Autodesk Inventor part; units mm, degrees
ref_plane "YZ Plane" through (0, 0, 0) normal (1, 0, 0) x (0, 1, 0)
ref_plane "XZ Plane" through (0, 0, 0) normal (0, 1, 0) x (-1, 0, 0)
ref_plane "XY Plane" through (0, 0, 0) normal (0, 0, 1) x (1, 0, 0)
sketch "Sketch1" plane through (0, 0, 0) normal (0, 0, 1) x (1, 0, 0)
  line L0 (-96.7048, 41.9035) -> (-96.7048, -42.0965)
  line L1 (-96.7048, -42.0965) -> (-72.3448, -42.0965)
  line L2 (-72.3448, -42.0965) -> (-72.3448, -36.0115)
  line L3 (-72.3448, -36.0115) -> (-48.7048, -36.0115)
  line L4 (-48.7048, -36.0115) -> (-48.7048, -42.0965)
  line L5 (-48.7048, -42.0965) -> (-24.3448, -42.0965)
  line L6 (-0.7048, -42.0965) -> (23.6552, -42.0965)
  line L7 (47.2952, -42.0965) -> (71.6552, -42.0965)
  line L8 (71.6552, -42.0965) -> (71.6552, -36.0115)
  line L9 (71.6552, -36.0115) -> (95.2952, -36.0115)
  line L10 (95.2952, -36.0115) -> (95.2952, 35.8185)
  line L11 (95.2952, 35.8185) -> (71.6552, 35.8185)
  line L12 (71.6552, 35.8185) -> (71.6552, 41.9035)
  line L13 (71.6552, 41.9035) -> (47.2952, 41.9035)
  line L14 (47.2952, 41.9035) -> (47.2952, 35.8185)
  line L15 (47.2952, 35.8185) -> (23.6552, 35.8185)
  line L16 (23.6552, 35.8185) -> (23.6552, 41.9035)
  line L17 (23.6552, 41.9035) -> (-0.7048, 41.9035)
  line L18 (-0.7048, 41.9035) -> (-0.7048, 35.8185)
  line L19 (-0.7048, 35.8185) -> (-24.3448, 35.8185)
  line L20 (-24.3448, 35.8185) -> (-24.3448, 41.9035)
  line L21 (-24.3448, 41.9035) -> (-48.7048, 41.9035)
  line L22 (-48.7048, 41.9035) -> (-48.7048, 35.8185)
  line L23 (-48.7048, 35.8185) -> (-72.3448, 35.8185)
  line L24 (-72.3448, 35.8185) -> (-72.3448, 41.9035)
  line L25 (-72.3448, 41.9035) -> (-96.7048, 41.9035)
  line L26 (-24.3448, -42.0965) -> (-24.3448, -36.0115)
  line L27 (-24.3448, -36.0115) -> (-0.7048, -36.0115)
  line L28 (-0.7048, -36.0115) -> (-0.7048, -42.0965)
  line L29 (23.6552, -42.0965) -> (23.6552, -36.0115)
  line L30 (23.6552, -36.0115) -> (47.2952, -36.0115)
  line L31 (47.2952, -36.0115) -> (47.2952, -42.0965)
  point P0 (0, 0)
  dimension "d0" = 84
  dimension "d1" = 24.36
  dimension "d2" = 23.64
  dimension "d3" = 24.36
  dimension "d5" = 24.36
  dimension "d8" = 23.64
  dimension "d9" = 71.83
  dimension "d10" = 23.64
  dimension "d11" = 6.085
  dimension "d12" = 6.085
  dimension "d13" = 6.085
  dimension "d14" = 24.36
  dimension "d15" = 23.64
  dimension "d16" = 24.36
  dimension "d17" = 23.64
  dimension "d18" = 24.36
  dimension "d19" = 23.64
  dimension "d20" = 24.36
  dimension "d21" = 23.64
  dimension "d22" = 23.64
extrude "Extrusion1" add sketch "Sketch1" against normal blind 3.25
sketch "Sketch2" plane through (0, 0, 0) normal (0, 0, 1) x (1, 0, 0)
  line L0 (-92.5348, 22.4285) -> (-92.5348, -22.6215)
  line L1 (-92.5348, -22.6215) -> (-88.4348, -22.6215)
  line L2 (-88.4348, -22.6215) -> (-88.4348, 22.4285)
  line L3 (-88.4348, 22.4285) -> (-92.5348, 22.4285)
  line L4 (-96.7048, 41.9035) -> (-96.7048, -42.0965)
  line L5 (-72.3448, 41.9035) -> (-96.7048, 41.9035)
  line L6 (-85.7648, 13.0835) -> (-85.7648, -13.2765)
  line L7 (-85.7648, -13.2765) -> (-58.5248, -13.2765)
  line L8 (-58.5248, -13.2765) -> (-58.5248, 13.0835)
  line L9 (-58.5248, 13.0835) -> (-85.7648, 13.0835)
  line L10 (-54.5548, 31.9735) -> (-54.5548, -32.1665)
  line L11 (-54.5548, -32.1665) -> (-41.9148, -32.1665)
  line L12 (-41.9148, -32.1665) -> (-41.9148, 31.9735)
  line L13 (-41.9148, 31.9735) -> (-54.5548, 31.9735)
  line L14 (-24.3448, 41.9035) -> (-48.7048, 41.9035)
  line L15 (-29.3448, 21.4335) -> (-29.3448, -21.6265)
  line L16 (-29.3448, -21.6265) -> (65.1152, -21.6265)
  line L17 (65.1152, -21.6265) -> (65.1152, 21.4335)
  line L18 (65.1152, 21.4335) -> (-29.3448, 21.4335)
  line L19 (73.8852, 31.9735) -> (73.8852, -32.1665)
  line L20 (73.8852, -32.1665) -> (86.5252, -32.1665)
  line L21 (86.5252, -32.1665) -> (86.5252, 31.9735)
  line L22 (71.6552, 35.8185) -> (95.2952, 35.8185)
  line L23 (86.5252, 31.9735) -> (73.8852, 31.9735)
  line L24 (95.2952, -36.0115) -> (95.2952, 35.8185)
  point P0 (0, 0)
  dimension "d25" = 4.17
  dimension "d26" = 4.1
  dimension "d27" = 45.05
  dimension "d28" = 19.475
  dimension "d29" = 10.94
  dimension "d30" = 26.36
  dimension "d31" = 27.24
  dimension "d32" = 42.15
  dimension "d33" = 28.82
  dimension "d34" = 64.14
  dimension "d35" = 12.64
  dimension "d36" = 9.93
  dimension "d37" = 67.36
  dimension "d38" = 43.06
  dimension "d39" = 94.46
  dimension "d40" = 20.47
  dimension "d41" = 64.14
  dimension "d42" = 12.64
  dimension "d43" = 3.845
  dimension "d44" = 8.77
extrude "Extrusion2" cut sketch "Sketch2" against normal blind 4
sketch "Sketch3" plane through (0, 0, 0) normal (0, 0, 1) x (1, 0, 0)
  line L0 (-121.7905, 18.4035) -> (-90.4348, 18.4035)
  line L1 (-90.4348, 18.4035) -> (-90.4348, -18.5965)
  line L2 (-88.4348, 22.4285) -> (-88.4348, -22.6215)
  line L3 (-90.4348, -18.5965) -> (-121.7905, -18.5965)
  line L4 (-121.7905, -18.5965) -> (-121.7905, 18.4035)
  line L5 (-72.3448, 41.9035) -> (-96.7048, 41.9035)
  point P0 (0, 0)
  dimension "d47" = 37
  dimension "d48" = 23.5
  dimension "d49" = 2
extrude "Extrusion3" cut sketch "Sketch3" against normal blind 4
sketch "Sketch9" plane through (0, 0, 0) normal (0, 0, 1) x (1, 0, 0)
  line L0 (-92.5348, 28.4035) -> (-92.5348, -28.5965)
  line L1 (-92.5348, -28.5965) -> (-159.1348, -28.5965)
  line L2 (-159.1348, -28.5965) -> (-159.1348, 28.4035)
  line L3 (-159.1348, 28.4035) -> (-92.5348, 28.4035)
  line L4 (-92.5348, 18.4035) -> (-92.5348, 22.4285)
  line L5 (-72.3448, 41.9035) -> (-96.7048, 41.9035)
  line L6 (-96.7048, -42.0965) -> (-72.3448, -42.0965)
  point P0 (0, 0)
  dimension "d64" = 0
  dimension "d65" = 13.5
  dimension "d66" = 13.5
  dimension "d67" = 66.6
extrude "Extrusion6" add sketch "Sketch9" against normal blind 11.25
sketch "Sketch10" plane through (-159.1348, -28.5965, 0) normal (-1, 0, 0) x (0, 0, 1)
  circle A0 centre (9.5, 28.5) radius 18.5
  line L0 (0, 70.5) -> (-3.25, 70.5)
  line L1 (-11.25, 0) -> (-11.25, 57)
  point P0 (0, 28.5965)
  dimension "d70" = 42
  dimension "d71" = 37
  dimension "d72" = 20.75
extrude "Extrusion7" cut sketch "Sketch10" against normal blind 66.6
sketch "Sketch11" plane through (0, 0, 0) normal (0, 0, 1) x (1, 0, 0)
  point P0 (0, 0)
sketch "Sketch12" plane through (0, 0, 0) normal (0, 0, 1) x (1, 0, 0)
  line L0 (86.5252, 35.8185) -> (86.5252, -36.0115)
  line L1 (86.5252, -36.0115) -> (95.2952, -36.0115)
  line L2 (95.2952, -36.0115) -> (95.2952, 35.8185)
  line L3 (95.2952, 35.8185) -> (86.5252, 35.8185)
  line L4 (95.2952, -36.0115) -> (95.2952, 35.8185)
  line L5 (95.2952, 35.8185) -> (71.6552, 35.8185)
  line L6 (86.5252, 31.9735) -> (86.5252, -32.1665)
  line L7 (71.6552, -36.0115) -> (95.2952, -36.0115)
  line L8 (-41.9148, 12.1175) -> (-41.9148, 35.8185)
  line L9 (-41.9148, 35.8185) -> (-41.9148, -36.0115)
  line L10 (-41.9148, -36.0115) -> (-29.3448, -36.0115)
  line L11 (-41.9148, 31.9735) -> (-41.9148, -32.1665)
  line L12 (-29.3448, -36.0115) -> (-29.3448, 35.8185)
  line L13 (-29.3448, -21.6265) -> (-29.3448, 21.4335)
  line L14 (-29.3448, 35.8185) -> (-41.9148, 35.8185)
  line L15 (-0.7048, 35.8185) -> (-24.3448, 35.8185)
  line L16 (-24.3448, -36.0115) -> (-0.7048, -36.0115)
  point P0 (0, 0)
  dimension "d75" = 0
  dimension "d76" = 0
  dimension "d77" = 0
  dimension "d78" = 0
  dimension "d79" = 0
  dimension "d80" = 0
  dimension "d81" = 0
  dimension "d82" = 0
extrude "Extrusion8" add sketch "Sketch12" against normal blind 11.25
properties part number "new base"
Design review of the part built by this model. Coordinates are the model's own, in mm. A direction names the side the tool comes from. Give positions to 0.01 mm unless a question says otherwise; leave off trailing zeros. Write each loop counter-clockwise with the first axis right and the second up, starting at its lowest first coordinate (ties: lowest second). Pieces come first, ordered by that corner, then holes. Notation, with made-up numbers: (-16, 77.5) - (12, 77.5) arc R25 ccw to (12, 99.5) - close; hole circle Ø5 at (21, -40). An arc over 180 degrees is marked (long way). Return JSON: item names as keys, results as strings. Group by question number.
(1) We need section B-B, the plane z = -7.25. Give the boundary of the cut face in (x, y).
(2) To check wall thickness, follow probe 1 along X at (y, z) = (11.5, -2.75); probe 2 along X at (y, z) = (20, -2.25); probe 3 along X at (y, z) = (28, -5.5). State the ranges of each line that lie inside material, in increasing order.
(3) We need section A-A, the plane x = -17. Give the boundary of the cut face in (y, z), then the cut area to 3 significant figures.
(4) Machinability: for faces 5 (the cylindrical face through (-126, 0, -9)), 6 (the flat face through (-36, -36.012, -7)), 7 (the flat face through (86, 35.818, -3)), which of the approach directions +Z, -Z, +X, -X, +Y, -Y give a long, thin tool a straight path to every point of the face, cutting with its end or side? Answer none if there is none.
(5) We need section C-C, the plane y = -4. Give the boundary of the cut face in (x, z), then the cut area to 3 significant figures.
(6) Mouldability with a two-part tool opening along X and no side actions: class faces 1 (the flat face through (-27, 28, -3.25)), 2 (the flat face through (-159.135, -0.5, -9.3)), 3 (the flat face through (-41.915, -1, -6)), 4 (the flat face through (-125, -28.596, -6)) as +X half, -X half, draft (parallel to the pull), parting line (faces both ways), or undercut.
(7) We need section D-D, the plane x = -135.5. Give the boundary of the cut face in (y, z), then the cut area to 3 significant figures.
(8) Insertion check: pin 1 (1 mm diameter, centred on x = -71.5, z = -1.5, fed in from +Y); pin 2 (1.6 mm diameter, centred on y = -35.5, z = -2, fed in from -X); pin 3 (3.5 mm diameter, centred on y = -40.5, z = -1, fed in from +X). Each pin has a flat end and moves straight along its axis. Give the tip position at first contact, or say it passes through.
Reported:
{
 "1": {"outline": "(-159.13, -28.6) - (-92.53, -28.6) - (-92.53, -7.95) - (-159.13, -7.95) - close; (-159.13, 7.76) - (-92.53, 7.76) - (-92.53, 28.4) - (-159.13, 28.4) - close; (-41.91, -36.01) - (-29.34, -36.01) - (-29.34, 35.82) - (-41.91, 35.82) - close; (86.53, -36.01) - (95.3, -36.01) - (95.3, 35.82) - (86.53, 35.82) - close"},
 "2": {"probe 1": "x = -88.43 to -85.76, -58.52 to -54.55, -41.91 to -29.34, 65.12 to 73.89, 86.53 to 95.3", "probe 2": "x = -159.13 to -92.53, -88.43 to -54.55, -41.91 to -29.34, 65.12 to 73.89, 86.53 to 95.3", "probe 3": "x = -159.13 to -92.53, -41.91 to -29.34, 86.53 to 95.3"},
 "3": {"outline": "(-36.01, -3.25) - (-21.63, -3.25) - (-21.63, 0) - (-36.01, 0) - close; (21.43, -3.25) - (35.82, -3.25) - (35.82, 0) - (21.43, 0) - close", "area": "93.5 mm2"},
 "4": {"face 5": "+Z, -X", "face 6": "-Z, +X, -X, -Y", "face 7": "+Z, -Z, +X, +Y"},
 "5": {"outline": "(-159.13, -11.25) - (-92.53, -11.25) - (-92.53, -8.58) - (-159.13, -8.58) - close; (-88.43, -3.25) - (-85.76, -3.25) - (-85.76, 0) - (-88.43, 0) - close; (-58.52, -3.25) - (-54.55, -3.25) - (-54.55, 0) - (-58.52, 0) - close; (-41.91, -11.25) - (-29.34, -11.25) - (-29.34, 0) - (-41.91, 0) - close; (65.12, -3.25) - (73.89, -3.25) - (73.89, 0) - (65.12, 0) - close; (86.53, -11.25) - (95.3, -11.25) - (95.3, 0) - (86.53, 0) - close", "area": "468 mm2"},
 "6": {"face 1": "undercut", "face 2": "-X half", "face 3": "undercut", "face 4": "draft"},
 "7": {"outline": "(-28.6, -11.25) - (28.4, -11.25) - (28.4, 0) - (15.78, 0) arc R18.5 cw to (-15.97, 0) - (-28.6, 0) - close", "area": "439 mm2"},
 "8": {"pin 1": "stops at y = 35.82", "pin 2": "stops at x = -96.7", "pin 3": "stops at x = 71.66"}
}
